Work out the finished part from the listing and answer in its coordinate system (mm). Face numbers are marked on the shaded views. A direction names the side the tool comes from. Round coordinates to 2 decimals unless told otherwise and drop trailing zeros. Write each loop counter-clockwise with the first axis right and the second up, starting at its lowest first coordinate (ties: lowest second). Pieces come first, ordered by that corner, then holes.
1. Flat-ended cylindrical pins translate along their axes: pin 1 Ø8 at (y, z) = (-28, 5) entering from -X; pin 2 Ø6 at (x, z) = (11, 10) entering from +Y; pin 3 Ø4 at (x, z) = (-1.5, 9) entering from -Y. Find the tip coordinate at first contact, or state that the pin passes through.
2. A tool of negligible diameter and unlimited length cuts with its end or side. For the marked faces 1, 2 and 3, from which of +Z, -Z, +X, -X, +Y, -Y can it reach the whole face along a straight path? Write none if from no direction.
3. Find section A-A (y = 0). Write down the section's boundary in (x, z).
4. Find section C-C (x = 6). Count the separate pieces of the cut face and the enclosed holes in it, and give its area (3 significant figures).
5. Find section B-B (z = 7). Write down the section's boundary in (x, y), and give its area (3 significant figures).
6. Straight lines are drawn through the part: probe 1 along X at (y, z) = (9, 4.5); probe 2 along X at (y, z) = (7, 10); probe 3 along Z at (x, y) = (-17, 10). For each, find the intervals that lie inside material, in ascending order.
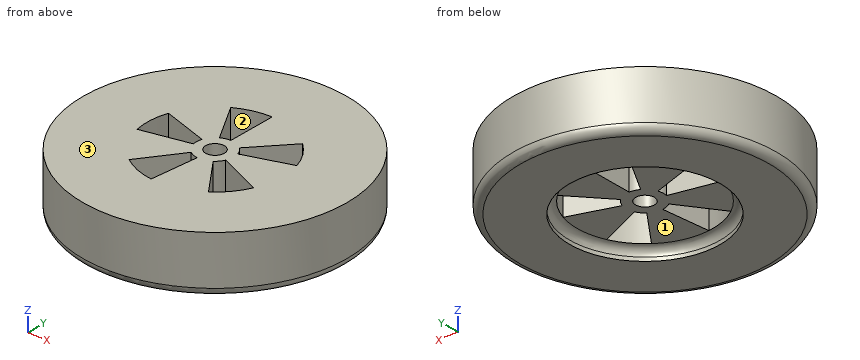
```python
from build123d import *

# Parameters (mm, degrees)
SKETCH1_R           = 35
BOSS_EXTRUDE1_DEPTH = 15
SKETCH2_R           = 20
CUT_EXTRUDE1_DEPTH  = 3
FILLET1_R           = 2
FILLET2_R           = 2
SKETCH4_R           = 2.5
CUT_EXTRUDE2_DEPTH  = 51.931326382
CUT_EXTRUDE3_DEPTH  = 51.931326382


with BuildPart() as part:
    # Sketch1 → Boss-Extrude1 (new body)
    with BuildSketch(Plane.XY):
        Circle(SKETCH1_R)
    extrude(amount=BOSS_EXTRUDE1_DEPTH)

    # Sketch2 → Cut-Extrude1 (cut)
    with BuildSketch(Plane(origin=(0, 0, 0), x_dir=(-1, 0, 0), z_dir=(0, 0, -1))):
        Circle(SKETCH2_R)
    extrude(amount=-CUT_EXTRUDE1_DEPTH, mode=Mode.SUBTRACT)

    # Fillet1
    fillet1_edges = [part.edges().sort_by_distance(p)[0] for p in [
        (-35, 0, 0),
    ]]
    fillet(fillet1_edges, radius=FILLET1_R)

    # Fillet2
    fillet2_edges = [part.edges().sort_by_distance(p)[0] for p in [
        (20, 0, 3),
    ]]
    fillet(fillet2_edges, radius=FILLET2_R)

    # Sketch4 → Cut-Extrude2 (cut, through all)
    with BuildSketch(Plane(origin=(0, 0, 3), x_dir=(-1, 0, 0), z_dir=(0, 0, -1))):
        Circle(SKETCH4_R)
    extrude(amount=-CUT_EXTRUDE2_DEPTH, mode=Mode.SUBTRACT)

    # Sketch5 → Cut-Extrude3 (cut, through all)
    with BuildSketch(Plane(origin=(0, 0, 3), x_dir=(-1, 0, 0), z_dir=(0, 0, -1))):
        with BuildLine():
            Line((0, 5), (0, 18))
            ThreePointArc((0, 18), (4.658742812, 17.386664873), (9, 15.588457268))
            Line((9, 15.588457268), (2.5, 4.330127019))
            ThreePointArc((2.5, 4.330127019), (1.294095226, 4.829629131), (0, 5))
        make_face()
        with BuildLine():
            Line((4.890738004, -1.039558454), (17.606656813, -3.742410435))
            ThreePointArc((17.606656813, -3.742410435), (17.975331626, 0.942047212), (17.119017293, 5.562305899))
            Line((17.119017293, 5.562305899), (4.755282581, 1.545084972))
            ThreePointArc((4.755282581, 1.545084972), (4.993147674, 0.261679781), (4.890738004, -1.039558454))
        make_face()
        with BuildLine():
            Line((0.522642316, -4.972609477), (1.881512339, -17.901394117))
            ThreePointArc((1.881512339, -17.901394117), (6.450623092, -16.804447677), (10.580134541, -14.562305899))
            Line((10.580134541, -14.562305899), (2.938926261, -4.045084972))
            ThreePointArc((2.938926261, -4.045084972), (1.791839748, -4.667902132), (0.522642316, -4.972609477))
        make_face()
        with BuildLine():
            Line((-4.567727288, -2.033683215), (-16.443818238, -7.321259575))
            ThreePointArc((-16.443818238, -7.321259575), (-13.988627306, -11.327767039), (-10.580134541, -14.562305899))
            Line((-10.580134541, -14.562305899), (-2.938926261, -4.045084972))
            ThreePointArc((-2.938926261, -4.045084972), (-3.885729807, -3.146601955), (-4.567727288, -2.033683215))
        make_face()
        with BuildLine():
            Line((-3.345653032, 3.715724127), (-12.044350914, 13.376606859))
            ThreePointArc((-12.044350914, 13.376606859), (-15.096070223, 9.80350263), (-17.119017293, 5.562305899))
            Line((-17.119017293, 5.562305899), (-4.755282581, 1.545084972))
            ThreePointArc((-4.755282581, 1.545084972), (-4.19335284, 2.723195175), (-3.345653032, 3.715724127))
        make_face()
    extrude(amount=-CUT_EXTRUDE3_DEPTH, mode=Mode.SUBTRACT)


solid = part.part
```
Worked answers:
1. pin 1: stops at x = -25.48
1. pin 2: stops at y = 34.07
1. pin 3: stops at y = -35
2. face 1: -Z
2. face 2: +Z, -Z
2. face 3: +Z, +X, -X, +Y, -Y
3. outline: (-35, 2) arc R2 ccw to (-33, 0) - (-20, 0) - (-20, 1) arc R2 cw to (-18, 3) - (-18, 15) - (-35, 15) - close; (-5, 3) - (-2.5, 3) - (-2.5, 15) - (-5, 15) - close; (2.5, 3) - (18, 3) arc R2 cw to (20, 1) - (20, 0) - (33, 0) arc R2 ccw to (35, 2) - (35, 15) - (2.5, 15) - close
4. separate pieces: 3
4. enclosed holes: 0
4. area: 796 mm2
5. outline: circle Ø70 at (0, 0); hole (-17.61, -3.74) - (-4.89, -1.04) arc R5 cw to (-4.76, 1.55) - (-17.12, 5.56) arc R18 ccw to start; hole (-10.58, -14.56) arc R18 ccw to (-1.88, -17.9) - (-0.52, -4.97) arc R5 cw to (-2.94, -4.05) - close; hole (-9, 15.59) - (-2.5, 4.33) arc R5 cw to (0, 5) - (0, 18) arc R18 ccw to start; hole circle Ø5 at (0, 0); hole (2.94, -4.05) - (10.58, -14.56) arc R18 ccw to (16.44, -7.32) - (4.57, -2.03) arc R5 cw to start; hole (3.35, 3.72) arc R5 cw to (4.76, 1.55) - (17.12, 5.56) arc R18 ccw to (12.04, 13.38) - close
5. area: 3,440 mm2
6. probe 1: x = -33.82 to -5.2, 0 to 8.1, 15.59 to 33.82
6. probe 2: x = -34.29 to -4.04, 0 to 6.3, 16.58 to 34.29
6. probe 3: z = 2.02 to 15
